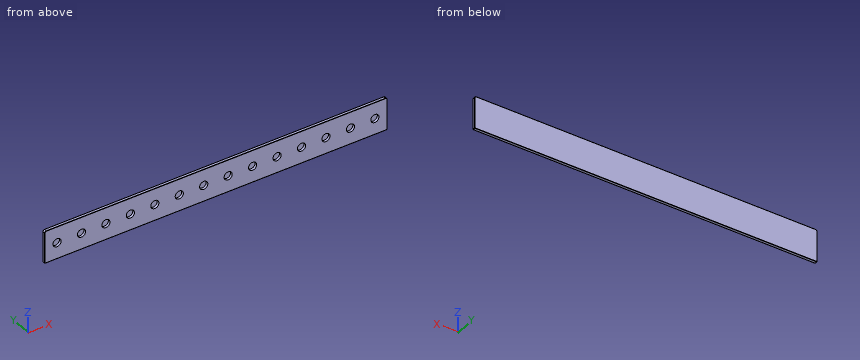
Autodesk Inventor part; units mm, degrees
ref_plane "Work Plane1" through (-210, 0.3, -39.7) normal (1, 0, 0) x (0, 0, -1)
ref_plane "YZ Plane" through (0, 0, 0) normal (1, 0, 0) x (0, 1, 0)
ref_plane "XZ Plane" through (0, 0, 0) normal (0, 1, 0) x (-1, 0, 0)
sketch "Sketch1" plane through (0, 0, 0) normal (0, 1, 0) x (-1, 0, 0)
  line L0 (0, 0) -> (420, 0)
  line L1 (420, 0) -> (420, -40)
  line L2 (420, -40) -> (0, -40)
  line L3 (0, -40) -> (0, 0)
  dimension "d0" = 420
  dimension "d1" = 40
extrude "Extrusion1" add sketch "Sketch1" along normal blind 3.5
fillet "Fillet1" radius 0.3 10 edges at (-210, 3.5, 0) (-210, 0, 0) (0, 0, -20) (0, 3.5, -20) (0, 1.75, -40) (-210, 3.5, -40) (-210, 0, -40) (-420, 0, -20) (-420, 1.75, -40) (-420, 3.5, -20)
sketch "Sketch2" plane through (0, 0, 0) normal (0, -1, 0) x (1, 0, 0)
  line L0 (-419.7, -39.7) -> (-419.7, -0.3)
  line L1 (-419.7, -20) -> (0, -20)
  circle A0 centre (-405, -20) radius 5
  circle A1 centre (-375, -20) radius 5
  circle A2 centre (-345, -20) radius 5
  circle A3 centre (-315, -20) radius 5
  line L2 (-420, 0) -> (-420, -39.7)
  line L3 (-315, -20) -> (-315, -8.0411)
  line L4 (-210.3, -20) -> (-630, -20)
  circle A4 centre (-225, -20) radius 5
  circle A5 centre (-255, -20) radius 5
  circle A6 centre (-285, -20) radius 5
  point P0 (0, 0)
  point P1 (-420, -0.3)
  dimension "d5" = 10
  dimension "d6" = 10
  dimension "d7" = 10
  dimension "d8" = 10
  dimension "d9" = 15
  dimension "d10" = 30
  dimension "d11" = 30
  dimension "d12" = 30
ref_plane "Work Plane1" through (-210, 0.3, -39.7) normal (1, 0, 0) x (0, 0, -1)
extrude "Extrusion2" cut sketch "Sketch2" against normal blind 3
mirror "Mirror1" about plane through (-210, 0.3, -39.7) normal (1, 0, 0) of "Extrusion2"
fillet "Fillet2" radius 2 6 edges at (-0.0879, 3.4121, -0.0879) (-0.0879, 0.0879, -0.0879) (0, 1.75, 0) (-419.9121, 3.4121, -0.0879) (-419.9121, 0.0879, -0.0879) (-420, 1.75, 0)
properties part number "LeftClamo"
The listing builds one solid part. Answer for the finished solid, in the listing's coordinates (mm). Give positions to 0.01 mm unless a question says otherwise; leave off trailing zeros. Order: outer loops, then holes, each group sorted by start corner. A loop starts at its lowest first (then second) coordinate and runs counter-clockwise, first axis right, second up. Notation, with made-up numbers: (-14, 81) - (14, 81) arc R14 ccw to (14, 87) - close; hole circle Ø8 at (87, 5). An arc over 180 degrees is marked (long way). Answer as CSV lines item,"result".
Q1. This flat-tipped pin is pushed along its axis until it touches: pin 1 Ø3 at (x, z) = (-283, -18) entering from -Y. Where does it stop, or does it pass through?
Answer key:
pin 1,"stops at y = 3"
Q2. A cutting plane is placed at B-B, the plane x = -195. Determine the outline of the cut face in (y, z).
Answer key:
outline,"(0, -39.7) arc R0.3 ccw to (0.3, -40) - (3.2, -40) arc R0.3 ccw to (3.5, -39.7) - (3.5, -0.3) arc R0.3 ccw to (3.2, 0) - (0.3, 0) arc R0.3 ccw to (0, -0.3) - (0, -15) - (3, -15) - (3, -25) - (0, -25) - close"
Q3. Straight lines are drawn through the part: L1, parallel to Z at x = -45, y = 1.25; L2, parallel to X at y = 0.25, z = -8; L3, parallel to Z at x = -107.5, y = 0.3. For each, find the intervals that lie inside material, in ascending order.
Answer key:
L1,"z = -40 to -25, -15 to 0"
L2,"x = -420 to 0"
L3,"z = -40 to -24.33, -15.67 to 0"
Q4. A cutting plane is placed at A-A, the plane y = 2.05. Count the separate pieces of the cut face and the enclosed holes in it, and give its area (3 significant figures).
Answer key:
separate pieces,"1"
enclosed holes,"14"
area,"15,700 mm^2"
Q5. A cutting plane is placed at C-C, the plane x = -74.5. Determine the outline of the cut face in (y, z), and give its area (3 significant figures).
Answer key:
outline,"(0, -39.7) arc R0.3 ccw to (0.3, -40) - (3.2, -40) arc R0.3 ccw to (3.5, -39.7) - (3.5, -0.3) arc R0.3 ccw to (3.2, 0) - (0.3, 0) arc R0.3 ccw to (0, -0.3) - (0, -15.03) - (3, -15.03) - (3, -24.97) - (0, -24.97) - close"
area,"110 mm^2"
